Autodesk Inventor part; units mm, degrees
ref_plane "YZ Plane" through (0, 0, 0) normal (1, 0, 0) x (0, 1, 0)
ref_plane "XZ Plane" through (0, 0, 0) normal (0, 1, 0) x (-1, 0, 0)
ref_plane "XY Plane" through (0, 0, 0) normal (0, 0, 1) x (1, 0, 0)
sketch "Эскиз1" plane through (0, 0, 0) normal (0, 1, 0) x (-1, 0, 0)
  line L0 (0, 0) -> (0, -70)
  line L1 (0, -70) -> (-9, -70)
  line L2 (-9, -70) -> (-9, -61)
  line L3 (-9, -61) -> (-176, -61)
  line L4 (-176, -61) -> (-194, -50)
  line L5 (-194, -50) -> (-194, 0)
  line L6 (-194, 0) -> (0, 0)
  point P0 (-4.5, -70)
  dimension "d0" = 194
  dimension "d1" = 9
  dimension "d14" = 140
  dimension "d103" = 122
  dimension "d104" = 100
  dimension "d105" = 18
revolve "Вращение1" add sketch "Эскиз1" angle 360 about axis through (194, 0, 0) along (-1, 0, 0)
sketch "Эскиз5" plane through (0, 0, 0) normal (0, 1, 0) x (-1, 0, 0)
  line L0 (-176, -61) -> (-176, 61)
  line L1 (-9, -61) -> (-9, 61)
  line L2 (-27, -40) -> (-107, -40)
  line L3 (-107, -40) -> (-107, 40)
  line L4 (-107, 40) -> (-27, 40)
  line L5 (-27, 40) -> (-27, -40)
  point P0 (0, 0)
  point P1 (-27, 0)
  point P2 (-9, 0)
  dimension "d38" = 80
  dimension "d40" = 18
extrude "Выдавливание4" add sketch "Эскиз5" along normal blind 110
sketch "Sketch15" plane through (27, 46.0543, 40) normal (0, 0, 1) x (1, 0, 0)
  circle A0 centre (22.5, 39.9457) radius 12.5
  circle A1 centre (57.5, 39.9457) radius 12.5
  line L0 (80, 63.9457) -> (0, 63.9457) construction
  line L1 (40, 63.9457) -> (40, 0) construction
  line L2 (0, 0) -> (80, 0) construction
  point P0 (-27, -46.0543)
  dimension "d106" = 25
  dimension "d107" = 35
  dimension "d108" = 24
extrude "Extrusion14" add sketch "Sketch15" along normal blind 25
fillet "Fillet1" radius 5 2 edges at (37, 86, 65) (72, 86, 65)
fillet "Fillet2" radius 2 8 edges at (27, 78.0272, 40) (67, 110, 40) (107, 78.0272, 40) (107, 110, 0) (67, 110, -40) (27, 110, 0) (107, 78.0272, -40) (27, 78.0272, -40)
sketch "Sketch16" plane through (9, 0, 0) normal (1, 0, 0) x (0, 0, -1)
  circle A0 centre (0, 0) radius 61
  line L0 (-38.8844, -47) -> (38.8844, -47)
  line L1 (0, -61) -> (0, -47) construction
  dimension "d113" = 14
extrude "Extrusion15" cut sketch "Sketch16" along normal up to surface (185 mm away) contours L0 A0 picked at (-10.0748, -48.9953)
sketch "Sketch17" plane through (9, -47, -38.8844) normal (0, -1, 0) x (1, 0, 0)
  line L0 (0, 77.7689) -> (167, 77.7689) construction
  line L1 (0, 0) -> (0, 77.7689) construction
  line L2 (167, 0) -> (0, 0) construction
  line L3 (185, 55.9432) -> (185, 21.8257) construction
  line L4 (19, -18.6156) -> (107, -18.6156)
  line L5 (107, -18.6156) -> (107, 96.3844)
  line L6 (107, 96.3844) -> (19, 96.3844)
  line L7 (19, 96.3844) -> (19, -18.6156)
  line L8 (19, -18.6156) -> (107, 96.3844) construction
  line L9 (107, -18.6156) -> (19, 96.3844) construction
  line L10 (28, 80.8844) -> (28, 83.8844) construction
  line L11 (25, 80.8844) -> (25, 83.8844)
  line L12 (31, 83.8844) -> (31, 80.8844)
  arc A0 (25, 80.8844) -> (31, 80.8844) centre (28, 80.8844) ccw
  arc A1 (31, 83.8844) -> (25, 83.8844) centre (28, 83.8844) ccw
  line L13 (98, 80.8844) -> (98, 83.8844) construction
  line L14 (101, 80.8844) -> (101, 83.8844)
  line L15 (95, 83.8844) -> (95, 80.8844)
  arc A2 (95, 80.8844) -> (101, 80.8844) centre (98, 80.8844) ccw
  arc A3 (101, 83.8844) -> (95, 83.8844) centre (98, 83.8844) ccw
  line L16 (98, -6.1156) -> (98, -3.1156) construction
  line L17 (101, -6.1156) -> (101, -3.1156)
  line L18 (95, -3.1156) -> (95, -6.1156)
  arc A4 (95, -6.1156) -> (101, -6.1156) centre (98, -6.1156) ccw
  arc A5 (101, -3.1156) -> (95, -3.1156) centre (98, -3.1156) ccw
  line L19 (28, -6.1156) -> (28, -3.1156) construction
  line L20 (31, -6.1156) -> (31, -3.1156)
  line L21 (25, -3.1156) -> (25, -6.1156)
  arc A6 (25, -6.1156) -> (31, -6.1156) centre (28, -6.1156) ccw
  arc A7 (31, -3.1156) -> (25, -3.1156) centre (28, -3.1156) ccw
  line L22 (-9, 108.8844) -> (-9, -31.1156)
  line L23 (63, 38.8844) -> (-9, 38.8844) construction
  point P0 (28, 82.3844)
  point P1 (98, 82.3844)
  point P2 (98, -4.6156)
  point P3 (28, -4.6156)
  dimension "d116" = 115
  dimension "d117" = 88
  dimension "d118" = 37
  dimension "d119" = 70
  dimension "d120" = 28
  dimension "d121" = 3
  dimension "d122" = 3
  dimension "d123" = 14
extrude "Extrusion16" add sketch "Sketch17" against normal blind 7
sketch "Sketch18" plane through (28, -47, 38.8844) normal (-1, 0, 0) x (0, 0, 1)
  line L0 (18.6156, 0) -> (18.6156, 7)
  line L1 (-96.3844, 0) -> (-96.3844, 7)
  line L2 (-96.3844, 7) -> (18.6156, 7)
  line L3 (-84.9388, 7) -> (-96.3844, 7)
  line L4 (18.6156, 7) -> (-1.3844, 7)
  line L5 (-1.3844, 7) -> (-1.3844, 17)
  line L6 (-1.3844, 17) -> (18.6156, 17)
  line L7 (18.6156, 17) -> (18.6156, 7)
  line L8 (-96.3844, 7) -> (-76.3844, 7)
  line L9 (-76.3844, 7) -> (-76.3844, 17)
  line L10 (-76.3844, 17) -> (-96.3844, 17)
  line L11 (-96.3844, 17) -> (-96.3844, 7)
  point P0 (-38.8844, 47)
  point P1 (-76.3844, 7)
  point P2 (-1.3844, 7)
  dimension "d126" = 20
  dimension "d127" = 10
extrude "Extrusion17" cut sketch "Sketch18" against normal blind 20
pattern_linear "Rectangular Pattern2" count 2 spacing 68 along (1, 0, 0) of "Extrusion17"
sketch "Sketch19" plane through (9, -47, -38.8844) normal (0, -1, 0) x (1, 0, 0)
  arc A0 (95, -6.1156) -> (101, -6.1156) centre (98, -6.1156) ccw
  line L0 (95, -6.1156) -> (95, -3.1156)
  arc A1 (101, -3.1156) -> (95, -3.1156) centre (98, -3.1156) ccw
  line L1 (101, -3.1156) -> (101, -6.1156)
  arc A2 (25, -6.1156) -> (31, -6.1156) centre (28, -6.1156) ccw
  line L2 (25, -6.1156) -> (25, -3.1156)
  arc A3 (31, -3.1156) -> (25, -3.1156) centre (28, -3.1156) ccw
  line L3 (31, -3.1156) -> (31, -6.1156)
  arc A4 (95, 80.8844) -> (101, 80.8844) centre (98, 80.8844) ccw
  line L4 (95, 80.8844) -> (95, 83.8844)
  arc A5 (101, 83.8844) -> (95, 83.8844) centre (98, 83.8844) ccw
  line L5 (101, 83.8844) -> (101, 80.8844)
  line L6 (31, 83.8844) -> (31, 80.8844)
  arc A6 (25, 80.8844) -> (31, 80.8844) centre (28, 80.8844) ccw
  line L7 (25, 80.8844) -> (25, 83.8844)
  arc A7 (31, 83.8844) -> (25, 83.8844) centre (28, 83.8844) ccw
  line L8 (0, 77.7689) -> (19, 77.7689)
  line L9 (0, 0) -> (0, 77.7689)
  line L10 (19, 0) -> (0, 0)
  line L11 (19, 0) -> (19, -18.6156)
  line L12 (19, -18.6156) -> (107, -18.6156)
  line L13 (107, -18.6156) -> (107, 0)
  line L14 (167, 0) -> (107, 0)
  line L15 (185, 55.9432) -> (185, 21.8257)
  line L16 (107, 77.7689) -> (167, 77.7689)
  line L17 (107, 77.7689) -> (107, 96.3844)
  line L18 (107, 96.3844) -> (19, 96.3844)
  line L19 (19, 96.3844) -> (19, 77.7689)
  point P0 (-9, 38.8844)
extrude "Extrusion18" cut sketch "Sketch19" against normal blind 10
equation "\"Reductor_angle\" = 180deg"
properties part number "СДР 060 Мотор-редуктор 2.0"
Build history of the part. All positions in model axes, mm. A direction names the side the tool comes from. Round coordinates to 2 decimals unless told otherwise and drop trailing zeros. Write each loop counter-clockwise with the first axis right and the second up, starting at its lowest first coordinate (ties: lowest second). Pieces come first, ordered by that corner, then holes. Notation, with made-up numbers: M 47.25,65.25 L 86.25,65.25 A21 ccw 86.25,96.25 Z; hole C 80.25,65.25 d2. An arc over 180 degrees is marked long. Answer in a Markdown table with one row per item.
1. Mould opens along Y. For faces 1 (the face through (73, -44, 57.5)), 2 (the face through (192.87, 50.65, 1.98)), 3 (the face through (38, -35, 37.5)) say: +Y half, -Y half, draft (parallel to the pull), parting line (faces both ways), or undercut.
Geometry check:
| item | result |
|---|---|
| face 1 | draft |
| face 2 | parting line |
| face 3 | undercut |
2. Saw through at C-C (y = 64). List the corners of the cut face in (x, z), and give its area (3 significant figures).
Geometry check:
| item | result |
|---|---|
| outline | M 0,-28.35 L 9,-28.35 L 9,28.35 L 0,28.35 Z; M 27,-38 A2 ccw 29,-40 L 105,-40 A2 ccw 107,-38 L 107,38 A2 ccw 105,40 L 29,40 A2 ccw 27,38 Z |
| area | 6,910 mm2 |
3. Which spindle directions (+Z, -Z, +X, -X, +Y, -Y) get a long thin tool onto all of the face, cutting with end or side? Do faces 4 (the face through (28, -44, -50)), 5 (the face through (37, -44, 39)), 6 (the face through (28, -35, -44)), 7 (the face through (106, -35, 37.5)). Say none if no direction does.
Geometry check:
| item | result |
|---|---|
| face 4 | -Z, -Y |
| face 5 | -Y |
| face 6 | -Z |
| face 7 | +Z |
4. Probe L1, parallel to X at y = 83.5, z = -23.5; L2, parallel to Y at x = 85.5, z = -24; L3, parallel to Z at x = 82, y = 101.5. List the from-to ranges inside material, lowest first. Write a range as [from, to].
Geometry check:
| item | result |
|---|---|
| L1 | [27, 107] |
| L2 | [-47, 110] |
| L3 | [-40, 40] |
5. Saw through at A-A (y = 0). List the corners of the cut face in (x, z), and give its area (3 significant figures).
Geometry check:
| item | result |
|---|---|
| outline | M 0,-70 L 9,-70 L 9,-61 L 176,-61 L 194,-50 L 194,50 L 176,61 L 9,61 L 9,70 L 0,70 Z |
| area | 23,600 mm2 |
6. Saw through at D-D (x = 66). List the corners of the cut face in (y, z).
Geometry check:
| item | result |
|---|---|
| outline | M -47,-57.5 L -40,-57.5 L -40,-46.05 A61 ccw 46.05,-40 L 108,-40 A2 ccw 110,-38 L 110,38 A2 ccw 108,40 L 46.05,40 A61 ccw -40,46.05 L -40,57.5 L -47,57.5 Z |
7. Saw through at B-B (z = 0). List the corners of the cut face in (x, y).
Geometry check:
| item | result |
|---|---|
| outline | M 0,-70 L 9,-70 L 9,-47 L 194,-47 L 194,50 L 176,61 L 107,61 L 107,108 A2 ccw 105,110 L 29,110 A2 ccw 27,108 L 27,61 L 9,61 L 9,70 L 0,70 Z |
8. Flat gauge pins, fed straight in: P1, Ø3.5, axis at y = -43, z = -43.5, coming from the +X side; P2, Ø5, axis at y = -33.5, z = 42.5, coming from the +X side; P3, Ø6, axis at x = 144.5, z = 50, coming from the +Y side. Where does each tip first touch, or does it go through?
Geometry check:
| item | result |
|---|---|
| P1 | x = 178.59 |
| P2 | x = 191.36 |
| P3 | y = 38.88 |
